Check sheet for the drawn part. Datum: minimum x, y, z corner. Units: mm. Round coordinates to 2 decimals unless told otherwise and drop trailing zeros. Write each loop counter-clockwise with the first axis right and the second up, starting at its lowest first coordinate (ties: lowest second). Pieces come first, ordered by that corner, then holes. Notation, with made-up numbers: (64, 10) -> (113, 10) arc R30 ccw to (113, 47) -> close; hole circle Ø5 at (88, -29.75). An arc over 180 degrees is marked (long way). One line per item, written item: value.
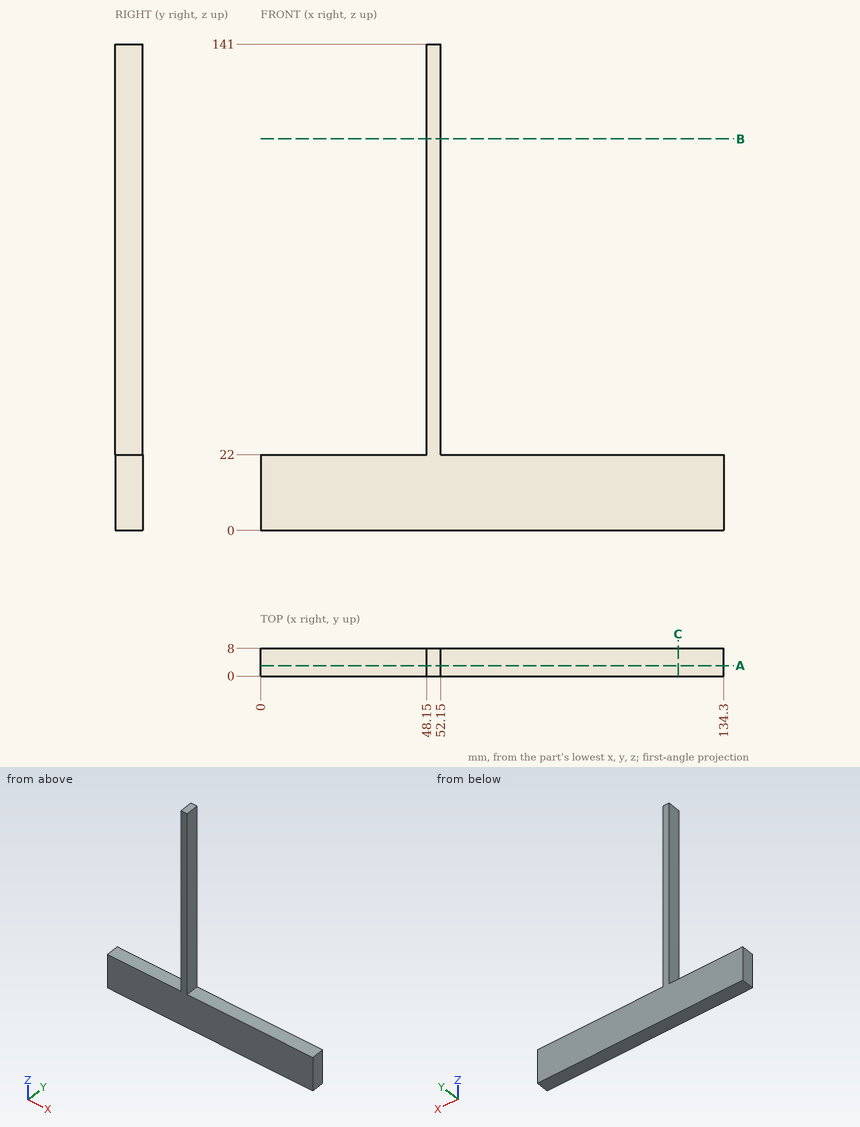
Item 1: Sectioned sample at C-C on x = 121. Enter the section's corners in (y, z).
Answer:
outline: (0, 0) -> (8, 0) -> (8, 22) -> (0, 22) -> close
Item 2: Depth check by flat-ended pin: P1, Ø3, axis at x = 98, y = 7, coming from the -Z side; P2, Ø2.5, axis at x = 74, y = 5, coming from the +Z side; P3, Ø2, axis at y = 7, z = 112.5, coming from the -X side; P4, Ø2.5, axis at y = 3, z = 95, coming from the +X side. Enter the tip coordinate at first touch or a pass-through.
Answer:
P1: stops at z = 0
P2: stops at z = 22
P3: stops at x = 48.15
P4: stops at x = 52.15
Item 3: Sectioned sample at A-A on y = 3. Enter the section's corners in (x, z).
Answer:
outline: (0, 0) -> (134.3, 0) -> (134.3, 22) -> (52.15, 22) -> (52.15, 141) -> (48.15, 141) -> (48.15, 22) -> (0, 22) -> close
Item 4: Sectioned sample at B-B on z = 113.5. Enter the section's corners in (x, y).
Answer:
outline: (48.15, 0) -> (52.15, 0) -> (52.15, 8) -> (48.15, 8) -> close
Item 5: Thickness scan on line 1 (Z direction, x = 119, y = 3.5); line 2 (X direction, y = 5.25, z = 124.5). Record the ranges inside material, lowest first.
Answer:
line 1: z = 0 to 22
line 2: x = 48.15 to 52.15
